Input: part model. Units: mm. Frame: model coordinates. A direction names the side the tool comes from. Give positions to 0.01 mm unless a question says otherwise; leave off trailing zeros. Write each loop counter-clockwise with the first axis right and the second up, starting at its lowest first coordinate (ties: lowest second). Pieces come first, ordered by that corner, then holes. Notation, with made-up numbers: (-12.5, 49) -> (20.5, 49) arc R5 cw to (20.5, 54) -> close; hole circle Ø11 at (17, 65.5). An arc over 180 degrees is marked (long way). Return JSON: item names as keys, results as strings. Group by question number.
Item 1: Pin query (flat end, axial travel): P1, Ø4, axis at x = 1, y = -1, coming from the +Z side; P2, Ø0.9, axis at x = -17.5, z = 2, coming from the -Y side; P3, Ø0.9, axis at y = 17, z = 1.5, coming from the -X side; P4, Ø0.9, axis at x = -4, z = 1.5, coming from the +Y side. Return the tip coordinate at first contact, or that it passes through.
Item 2: Section C-C, the plane z = 1.75. Return loops of the section in (x, y), then the cut area to 3 significant figures.
Item 3: Mould query, pull axis X, two halves, no side actions, for faces 6 (the face through (20.5, 0, 1)), 7 (the face through (0, -15.5, 1)), 8 (the face through (-13, -19, 1)). Classes: released by +X, released by -X, zero draft, split by the parting line, or undercut.
Item 4: Set-up query: faces 1 (the face through (0, 15.5, 1)), 2 (the face through (16.5, 17, 1)), 3 (the face through (-18, 15.5, 1)), 4 (the face through (-8.5, -17, 1)), 5 (the face through (18, -15.5, 1)). Return all of +Z, -Z, +X, -X, +Y, -Y with unobstructed straight access to the full face (end or side cutting, diameter ignored); none if empty.
Item 5: Section B-B, the plane x = 0. Return loops of the section in (y, z).
Item 6: Section A-A, the plane y = 0. Return loops of the section in (x, z).
Item 7: Line query: line 1 (X direction, y = 9, z = 1.35); line 2 (Y direction, x = 13, z = 0.5); line 3 (X direction, y = 16.5, z = 0.7). Output: solid intervals per line, ascending. Write a range as [from, to].
Item 8: Section D-D, the plane y = 9.5. Return loops of the section in (x, z), then the cut area to 3 significant figures.
from build123d import *

# Parameters (mm, degrees)
BOSS_EXTRUDE1_DEPTH          = 3
F_6_0_6_DIAMETER_HOLE1_D     = 6
F_6_0_6_DIAMETER_HOLE1_DEPTH = 3
M3_CLEARANCE_HOLE1_D         = 3.4
M3_CLEARANCE_HOLE1_DEPTH     = 3.001
MIRROR2_COPY_1_D             = 3.4
MIRROR2_COPY_1_DEPTH         = 3.001


with BuildPart() as part:
    # Sketch1 → Boss-Extrude1 (new body)
    with BuildSketch(Plane.XY):
        Polygon((20.5, -15.5), (20.5, 15.5), (16.5, 15.5), (16.5, 19), (8.5, 19), (8.5, 15.5), (-8.5, 15.5), (-8.5, 19), (-16.5, 19), (-16.5, 15.5), (-20.5, 15.5), (-20.5, -15.5), (-16.5, -15.5), (-16.5, -19), (-8.5, -19), (-8.5, -15.5), (8.5, -15.5), (8.5, -19), (16.5, -19), (16.5, -15.5), align=None)
    extrude(amount=BOSS_EXTRUDE1_DEPTH)

    # Ø6.0 (6) Diameter Hole1
    with Locations(Plane.XY.offset(3)):
        with Locations((0, 0)):
            Hole(F_6_0_6_DIAMETER_HOLE1_D / 2, depth=F_6_0_6_DIAMETER_HOLE1_DEPTH)

    # M3 Clearance Hole1
    with Locations(Plane.XY.offset(3)):
        with Locations((14.5, 9.5)):
            m3_clearance_hole1 = Hole(M3_CLEARANCE_HOLE1_D / 2, depth=M3_CLEARANCE_HOLE1_DEPTH)

    # Mirror1: M3 Clearance Hole1 across plane
    add(m3_clearance_hole1.mirror(Plane(origin=(0, 0, 0), x_dir=(0, 0, 1), z_dir=(1, 0, 0))), mode=Mode.SUBTRACT)

    # Mirror2: M3 Clearance Hole1 across plane
    add(m3_clearance_hole1.mirror(Plane.ZX), mode=Mode.SUBTRACT)

    # Mirror2 copy 1
    with Locations(Plane(origin=(0, 0, 3), x_dir=(-1, 0, 0), z_dir=(0, 0, 1))):
        with Locations((14.5, 9.5)):
            Hole(MIRROR2_COPY_1_D / 2, depth=MIRROR2_COPY_1_DEPTH)


solid = part.part
Answer below:
{
 "1": {"P1": "stops at z = 3", "P2": "stops at y = -15.5", "P3": "stops at x = -16.5", "P4": "stops at y = 15.5"},
 "2": {"outline": "(-20.5, -15.5) -> (-16.5, -15.5) -> (-16.5, -19) -> (-8.5, -19) -> (-8.5, -15.5) -> (8.5, -15.5) -> (8.5, -19) -> (16.5, -19) -> (16.5, -15.5) -> (20.5, -15.5) -> (20.5, 15.5) -> (16.5, 15.5) -> (16.5, 19) -> (8.5, 19) -> (8.5, 15.5) -> (-8.5, 15.5) -> (-8.5, 19) -> (-16.5, 19) -> (-16.5, 15.5) -> (-20.5, 15.5) -> close; hole circle Ø3.4 at (-14.5, -9.5); hole circle Ø3.4 at (-14.5, 9.5); hole circle Ø6 at (0, 0); hole circle Ø3.4 at (14.5, -9.5); hole circle Ø3.4 at (14.5, 9.5)", "area": "1,320 mm2"},
 "3": {"face 6": "released by +X", "face 7": "undercut", "face 8": "zero draft"},
 "4": {"face 1": "+Z, -Z, +Y", "face 2": "+Z, -Z, +X, +Y", "face 3": "+Z, -Z, -X, +Y", "face 4": "+Z, -Z, -Y", "face 5": "+Z, -Z, +X, -Y"},
 "5": {"outline": "(-15.5, 0) -> (-3, 0) -> (-3, 3) -> (-15.5, 3) -> close; (3, 0) -> (15.5, 0) -> (15.5, 3) -> (3, 3) -> close"},
 "6": {"outline": "(-20.5, 0) -> (-3, 0) -> (-3, 3) -> (-20.5, 3) -> close; (3, 0) -> (20.5, 0) -> (20.5, 3) -> (3, 3) -> close"},
 "7": {"line 1": "x = [-20.5, -16.12], [-12.88, 12.88], [16.12, 20.5]", "line 2": "y = [-19, -10.3], [-8.7, 8.7], [10.3, 19]", "line 3": "x = [-16.5, -8.5], [8.5, 16.5]"},
 "8": {"outline": "(-20.5, 0) -> (-16.2, 0) -> (-16.2, 3) -> (-20.5, 3) -> close; (-12.8, 0) -> (12.8, 0) -> (12.8, 3) -> (-12.8, 3) -> close; (16.2, 0) -> (20.5, 0) -> (20.5, 3) -> (16.2, 3) -> close", "area": "103 mm2"}
}
